Could you check a few things on this model? Use its own coordinates, in mm. Coordinates: 2 decimals unless noted, no trailing zeros. Loops run counter-clockwise (first coordinate to the right, second up) from the corner with the lowest first, then second, coordinate; pieces in that order, holes last.
from build123d import *

# Parameters (mm, degrees)
SKETCH019_W             = 47
SKETCH019_H             = 44
PAD004_DEPTH            = 2
SKETCH018_R             = 7
HOLE008_DEPTH           = 25
SKETCH017_R             = 1.8
HOLE007_DEPTH           = 25
FILLET002_R             = 2
BODY005_PLACEMENT_ANGLE = 180


with BuildPart() as part:
    # Sketch019 → Pad004 (new body)
    with BuildSketch(Plane.XY):
        Rectangle(SKETCH019_W, SKETCH019_H)
    extrude(amount=PAD004_DEPTH)

    # Sketch018 (on DatumPlane) → Hole008 (cut)
    with BuildSketch(Plane.XY.offset(2)):
        Circle(SKETCH018_R)
    extrude(amount=-HOLE008_DEPTH, mode=Mode.SUBTRACT)

    # Sketch017 (on DatumPlane) → Hole007 (cut)
    with BuildSketch(Plane.XY.offset(2)):
        with Locations((-16, 16)):
            Circle(SKETCH017_R)
        with Locations((16, 16)):
            Circle(SKETCH017_R)
        with Locations((-16, -16)):
            Circle(SKETCH017_R)
        with Locations((16, -16)):
            Circle(SKETCH017_R)
    extrude(amount=-HOLE007_DEPTH, mode=Mode.SUBTRACT)

    # Fillet002
    fillet002_edges = [part.edges().sort_by_distance(p)[0] for p in [
        (-23.5, -22, 1),
        (23.5, -22, 1),
        (23.5, 22, 1),
        (-23.5, 22, 1),
    ]]
    fillet(fillet002_edges, radius=FILLET002_R)


with BuildPart() as part_1:
    # Body005 placement: moved
    add(part.part.moved(Location((0, 0, 27))).rotate(Axis((0, 0, 27), (0, 0, 1)), BODY005_PLACEMENT_ANGLE))


solid = part_1.part
(1) Imagine slicing it at D-D, the plane z = 28.6. Write out the boundary of the cut face in (x, y).
Answers:
outline: (-23.5, -20) arc R2 ccw to (-21.5, -22) - (21.5, -22) arc R2 ccw to (23.5, -20) - (23.5, 20) arc R2 ccw to (21.5, 22) - (-21.5, 22) arc R2 ccw to (-23.5, 20) - close; hole circle Ø3.6 at (-16, -16); hole circle Ø3.6 at (-16, 16); hole circle Ø14 at (0, 0); hole circle Ø3.6 at (16, -16); hole circle Ø3.6 at (16, 16)
(2) For pin 1 (8.5 mm diameter, centred on x = 0, y = 0, fed in from +Z), with a flat end and sliding along its axis, tell me the tip position at first contact or that it passes through.
Answers:
pin 1: passes through
(3) Imagine slicing it at A-A, the plane x = 0. Write out the boundary of the cut face in (y, z), and give its area (3 significant figures).
Answers:
outline: (-22, 27) - (-7, 27) - (-7, 29) - (-22, 29) - close; (7, 27) - (22, 27) - (22, 29) - (7, 29) - close
area: 60.0 mm2
(4) I need wall thicknesses on probe 1 along Y at (x, z) = (16, 27.8); probe 2 along Y at (x, z) = (-15.5, 28.3); probe 3 along Y at (x, z) = (1.5, 27.3). Which ranges of each line are inside material? Lowest first, please.
Answers:
probe 1: y = -22 to -17.8, -14.2 to 14.2, 17.8 to 22
probe 2: y = -22 to -17.73, -14.27 to 14.27, 17.73 to 22
probe 3: y = -22 to -6.84, 6.84 to 22
(5) Imagine slicing it at B-B, the plane x = 16. Write out the boundary of the cut face in (y, z), and give its area (3 significant figures).
Answers:
outline: (-22, 27) - (-17.8, 27) - (-17.8, 29) - (-22, 29) - close; (-14.2, 27) - (14.2, 27) - (14.2, 29) - (-14.2, 29) - close; (17.8, 27) - (22, 27) - (22, 29) - (17.8, 29) - close
area: 73.6 mm2
(6) We'd pull the mould along Y, two halves only. Please class faces 1 (the face through (6, -5, 27)), 2 (the face through (-15.766, 14.215, 28.014)), 3 (the face through (-22.9, 21.43, 28.01)), 4 (the face through (-22.9, -21.43, 28.01)): +Y half, -Y half, draft (parallel to the pull), parting line (faces both ways), or undercut.
Answers:
face 1: draft
face 2: undercut
face 3: +Y half
face 4: -Y half
(7) Imagine slicing it at C-C, the plane y = -16. Write out the boundary of the cut face in (x, z), and give its area (3 significant figures).
Answers:
outline: (-23.5, 27) - (-17.8, 27) - (-17.8, 29) - (-23.5, 29) - close; (-14.2, 27) - (14.2, 27) - (14.2, 29) - (-14.2, 29) - close; (17.8, 27) - (23.5, 27) - (23.5, 29) - (17.8, 29) - close
area: 79.6 mm2
